For this review, take the finished solid that the model builds, in its own axes (mm). Coordinates: 2 decimals unless noted, no trailing zeros. Loops run counter-clockwise (first coordinate to the right, second up) from the corner with the lowest first, then second, coordinate; pieces in that order, holes last. Notation, with made-up numbers: (76.5, 38) -> (89.5, 38) arc R20 ccw to (89.5, 72) -> close; hole circle Ø8 at (11, 73). An arc over 180 degrees is marked (long way). Use a Markdown table: item, result.
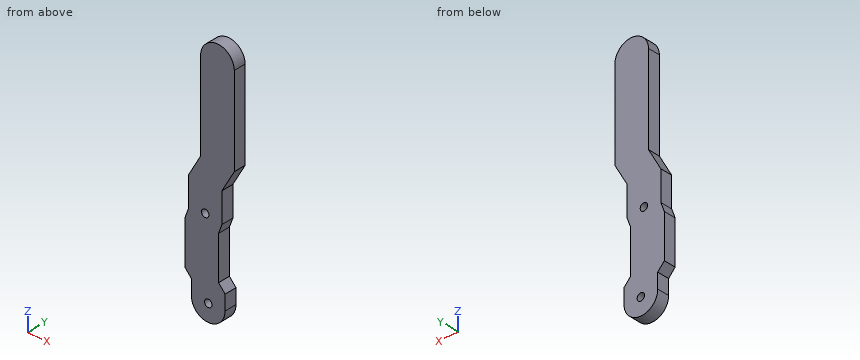
from build123d import *

# Parameters (mm, degrees)
F0_R     = 3
F1_DEPTH = 10


with BuildPart() as f1:
    # F0 (on Front) → F1 (new body)
    with BuildSketch(Plane.XZ):
        with BuildLine():
            ThreePointArc((-21.40014, 68.208159), (-35.014491, 81.592238), (-48.712137, 68.293419))
            Line((-48.712137, 68.293419), (-48.712137, -3.706581))
            Line((-48.712137, -3.706581), (-58.68246, -21.230183))
            Line((-58.68246, -21.230183), (-58.68246, -45.230183))
            Line((-58.68246, -45.230183), (-61.472507, -52.727892))
            Line((-61.472507, -52.727892), (-61.472507, -87.727892))
            Line((-61.472507, -87.727892), (-56.144382, -93.695394))
            Line((-56.144382, -93.695394), (-56.144382, -105.746023))
            ThreePointArc((-56.144382, -105.746023), (-42.531147, -119.487347), (-28.832385, -105.831283))
            Line((-28.832385, -105.831283), (-28.832385, -93.780654))
            Line((-28.832385, -93.780654), (-34.160511, -87.813152))
            Line((-34.160511, -87.813152), (-34.160511, -52.813152))
            Line((-34.160511, -52.813152), (-31.370464, -45.315443))
            Line((-31.370464, -45.315443), (-31.370464, -21.315443))
            Line((-31.370464, -21.315443), (-21.40014, -3.791841))
            Line((-21.40014, -3.791841), (-21.40014, 67.656904))
            Line((-21.40014, 67.656904), (-21.40014, 68.208159))
        make_face()
        with Locations((-42.488516, -105.831283)):
            Circle(F0_R, mode=Mode.SUBTRACT)
        with Locations((-44.960245, -42.831283)):
            Circle(F0_R, mode=Mode.SUBTRACT)
    extrude(amount=F1_DEPTH)


solid = f1.part
(1) Take a section at A-A on y = -8.25. Write out the cut boundary in (x, z), plus the area to 3 significant figures.
Found:
| item | result |
|---|---|
| outline | (-61.47, -87.73) -> (-56.14, -93.7) -> (-56.14, -105.75) arc R13.66 ccw (long way) to (-28.83, -105.83) -> (-28.83, -93.78) -> (-34.16, -87.81) -> (-34.16, -52.81) -> (-31.37, -45.32) -> (-31.37, -21.32) -> (-21.4, -3.79) -> (-21.4, 68.21) arc R13.66 ccw to (-48.71, 68.29) -> (-48.71, -3.71) -> (-58.68, -21.23) -> (-58.68, -45.23) -> (-61.47, -52.73) -> close; hole circle Ø6 at (-44.96, -42.83); hole circle Ø6 at (-42.49, -105.83) |
| area | 5,280 mm^2 |
(2) For line 1 along X through (y, z) = (-8.5, 17.5); line 2 along Z through (x, y) = (-41.5, -1); line 3 along Z through (x, y) = (-41, -0.5), list the stretches that pass through material, from the lowest coordinate up.
Found:
| item | result |
|---|---|
| line 1 | x = -48.71 to -21.4 |
| line 2 | z = -119.45 to -108.66, -103 to 79.98 |
| line 3 | z = -119.41 to -108.44, -103.23 to 80.23 |
(3) For pin 1 Ø5 at (y, z) = (-3, -65.5) entering from +X; pin 2 Ø5.5 at (x, z) = (-42.49, -105.83) entering from +Y; pin 3 Ø5 at (y, z) = (-2.5, -33) entering from +X, all flat-tipped, find the tip position at first contact; note any pin that passes through.
Found:
| item | result |
|---|---|
| pin 1 | stops at x = -34.16 |
| pin 2 | passes through |
| pin 3 | stops at x = -31.37 |
(4) Take a section at B-B on z = 12.5. Write out the cut boundary in (x, y).
Found:
| item | result |
|---|---|
| outline | (-48.71, -10) -> (-21.4, -10) -> (-21.4, 0) -> (-48.71, 0) -> close |
